```python
from build123d import *

# Parameters (mm, degrees)
RESSALTO_EXTRUS_O1_DEPTH = 15
ESBO_O3_R                = 1.5
CORTE_EXTRUS_O1_DEPTH    = 7
CORTE_EXTRUS_O2_DEPTH    = 2
FILETE1_R                = 1.5
FILETE2_R                = 2
FILETE3_R                = 5


# Some blends are built 0.0001 mm under size
with BuildPart() as part:
    # Esboço2 → Ressalto-extrusão1 (new body)
    with BuildSketch(Plane.XY):
        with BuildLine():
            Line((-25, -3), (-25, -10))
            Line((-25, -10), (25, -10))
            Line((25, -10), (25, -3))
            Line((25, -3), (9.369164851, -3))
            Line((9.369164851, -3), (9.369164851, -0.027094938))
            ThreePointArc((9.369164851, -0.027094938), (16.19072285, 11.863279554), (11.490485194, 24.740485194))
            Line((11.490485194, 24.740485194), (9.369164851, 22.619164851))
            ThreePointArc((9.369164851, 22.619164851), (0, 0), (-9.369164851, 22.619164851))
            Line((-9.369164851, 22.619164851), (-11.490485194, 24.740485194))
            ThreePointArc((-11.490485194, 24.740485194), (-16.19072285, 11.863279554), (-9.369164851, -0.027094938))
            Line((-9.369164851, -0.027094938), (-9.369164851, -3))
            Line((-9.369164851, -3), (-25, -3))
        make_face()
    extrude(amount=RESSALTO_EXTRUS_O1_DEPTH)

    # Esboço3 → Corte-extrusão1 (cut)
    with BuildSketch(Plane(origin=(0, -3, 0), x_dir=(1, 0, 0), z_dir=(0, 1, 0))):
        with Locations(Location((22, -7.5, 0), (0, 0, 270))):
            Circle(ESBO_O3_R)
        with Locations(Location((-22, -7.5, 0), (0, 0, 180))):
            Circle(ESBO_O3_R)
    extrude(amount=-CORTE_EXTRUS_O1_DEPTH, mode=Mode.SUBTRACT)

    # Esboço5 → Corte-extrusão2 (cut)
    with BuildSketch(Plane(origin=(0, -3, 0), x_dir=(1, 0, 0), z_dir=(0, 1, 0))):
        Polygon((22, -4.613248654), (19.5, -6.056624327), (19.5, -8.943375673), (22, -10.386751346), (24.5, -8.943375673), (24.5, -6.056624327), align=None)
        Polygon((-24.5, -6.056624327), (-22, -4.613248654), (-19.5, -6.056624327), (-19.5, -8.943375673), (-22, -10.386751346), (-24.5, -8.943375673), align=None)
    extrude(amount=-CORTE_EXTRUS_O2_DEPTH, mode=Mode.SUBTRACT)

    # Filete1
    filete1_edges = [part.edges().sort_by_distance(p)[0] for p in [
        (10.429825023, 23.679825023, 15),
        (-10.429825023, 23.679825023, 0),
        (0, 0, 0),
        (10.429825023, 23.679825023, 0),
        (0, 0, 15),
        (-11.490485194, 24.740485194, 7.5),
        (-9.369164851, 22.619164851, 7.5),
        (9.369164851, 22.619164851, 7.5),
        (11.490485194, 24.740485194, 7.5),
        (-10.429825023, 23.679825023, 15),
    ]]
    fillet(filete1_edges, radius=FILETE1_R - 0.0001)  # a hair under: the kernel refuses the full size

    # Filete2
    # the kernel refuses this fillet: 2 mm, written as the material it adds along each edge
    with BuildSketch(Plane(origin=(9.369164851, -0.027094938, 0), x_dir=(0.7999862174060132, 0.600018376352274, 0), z_dir=(0, 0, 1))) as filete2_piece_1:
        with BuildLine():
            CenterArc((1.000602329, -1.999158651), FILETE2_R, 91.661980606, 51.466805628)
            Line((-0.599370106, -0.799121898), (0, 0))
            ThreePointArc((0, 0), (0.471298198, -0.006835961), (0.942596397, 0))
        make_face()
    extrude(amount=15)
    with BuildSketch(Plane(origin=(9.369164851, -3, 0), x_dir=(0, 1, 0), z_dir=(0, 0, 1)), Plane(origin=(-9.369164851, -3, 0), x_dir=(-1, 0, 0), z_dir=(0, 0, 1))) as filete2_piece_2:
        with BuildLine():
            CenterArc((FILETE2_R, -FILETE2_R), FILETE2_R, 90, 90)
            Line((0, -FILETE2_R), (0, 0))
            Line((0, 0), (FILETE2_R, 0))
        make_face()
    extrude(amount=15)
    with BuildSketch(Plane(origin=(-9.369164851, -0.027094938, 0), x_dir=(-0.799986217406012, 0.6000183763522756, 0), z_dir=(0, 0, 1))) as filete2_piece_3:
        with BuildLine():
            CenterArc((1.000602329, 1.999158651), FILETE2_R, 216.871213766, 51.466805628)
            Line((-0.599370106, 0.799121898), (0, 0))
            ThreePointArc((0, 0), (0.471298198, 0.006835961), (0.942596397, 0))
        make_face()
    extrude(amount=15)

    # Filete3
    filete3_edges = [part.edges().sort_by_distance(p)[0] for p in [
        (25, -6.5, 0),
        (-25, -6.5, 0),
        (-25, -6.5, 15),
        (25, -6.5, 15),
    ]]
    fillet(filete3_edges, radius=FILETE3_R)


solid = part.part
```
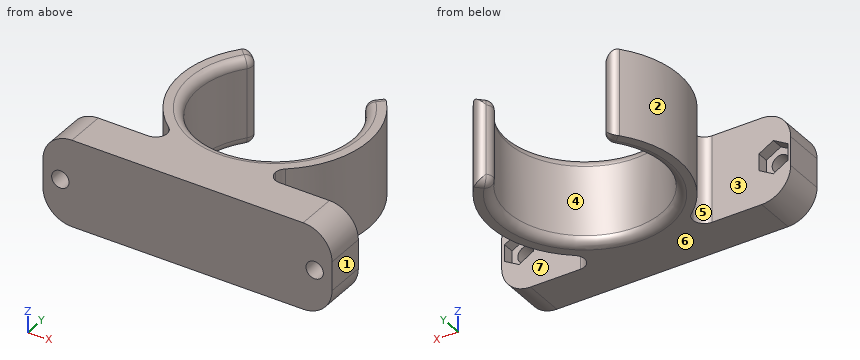
Geometry check sheet. Reference: the model listing, model coordinates, mm. Face numbers are marked on the shaded views. A direction names the side the tool comes from. Coordinates: 2 decimals unless noted, no trailing zeros. Loops run counter-clockwise (first coordinate to the right, second up) from the corner with the lowest first, then second, coordinate; pieces in that order, holes last.
Item 1: Access from +Z, -Z, +X, -X, +Y, -Y to the whole of each face (thin tool, end or side, straight path). Record for the marked faces 5, 6 and 7.
Item 2: Sectioned sample at B-B, the plane y = -8. Record the boundary of the cut face in (x, z), then the cut area to 3 significant figures.
Item 3: Release check for a two-part mould opening along X. For the marked faces 1, 2, 3 and 4 record: released by +X, released by -X, zero draft, split by the parting line, or undercut.
Item 4: Thickness scan on line 1 (X direction, y = -4.5, z = 7.25); line 2 (Y direction, x = 10.5, z = 12.75); line 3 (Y direction, x = 0, z = 5.25). Record the ranges inside material, lowest first.
Item 5: Sectioned sample at C-C, the plane z = 7.5. Count the separate pieces of the cut face and the enclosed holes in it, then the cut area to 3 significant figures.
Item 6: Go/stop test with flat-tipped pins: pin 1 Ø2.5 at (x, z) = (-22, 7.5) entering from +Y; pin 2 Ø5.5 at (x, z) = (-22.5, 8.5) entering from +Y; pin 3 Ø2.5 at (x, z) = (23, 7) entering from +Y. Record where each tip stops, or that it passes through.
Item 7: Sectioned sample at A-A, the plane x = -21. Record the boundary of the cut face in (y, z).
Item 8: Sectioned sample at D-D, the plane x = 0. Record the boundary of the cut face in (y, z), then the cut area to 3 significant figures.
Check result:
1. face 5: +Z, -Z, -X
1. face 6: -Z, +X, -X, +Y, -Y
1. face 7: +Z, -Z, +X
2. outline: (-25, 5) arc R5 ccw to (-20, 0) - (20, 0) arc R5 ccw to (25, 5) - (25, 10) arc R5 ccw to (20, 15) - (-20, 15) arc R5 ccw to (-25, 10) - close; hole circle Ø3 at (-22, 7.5); hole circle Ø3 at (22, 7.5)
2. area: 714 mm2
3. face 1: released by +X
3. face 2: released by -X
3. face 3: zero draft
3. face 4: undercut
4. line 1: x = -25 to -24.5, -19.5 to 19.5, 24.5 to 25
4. line 2: y = -10 to -2.8, 0.85 to 5.17, 21.33 to 23.74
4. line 3: y = -10 to 0
5. separate pieces: 3
5. enclosed holes: 0
5. area: 526 mm2
6. pin 1: passes through
6. pin 2: stops at y = -3
6. pin 3: stops at y = -5
7. outline: (-10, 0.1) - (-3, 0.1) - (-3, 5.19) - (-5, 5.19) - (-5, 6.38) - (-10, 6.38) - close; (-10, 8.62) - (-5, 8.62) - (-5, 9.81) - (-3, 9.81) - (-3, 14.9) - (-10, 14.9) - close
8. outline: (-10, 0) - (-1.5, 0) arc R1.5 ccw to (0, 1.5) - (0, 13.5) arc R1.5 ccw to (-1.5, 15) - (-10, 15) - close
8. area: 149 mm2
